from build123d import *

# Parameters (mm, degrees)
SKETCH_3_R          = 3
EXTRUDE_3_DEPTH     = 3
CUT_EXTRUDE_1_DEPTH = 232.050692133


with BuildPart() as part:
    # 草图3 → 凸台-拉伸3 (new body)
    with BuildSketch(Plane(origin=(0, 0, 0), x_dir=(1, 0, 0), z_dir=(0, 1, 0))):
        with BuildLine():
            Line((41.250352709, 37.437096955), (2.1711222, 37.437096955))
            ThreePointArc((2.1711222, 37.437096955), (-37.245354745, -4.362745688), (10.764053756, -35.921931278))
            Line((10.764053756, -35.921931278), (102.964763311, -8.293867902))
            ThreePointArc((102.964763311, -8.293867902), (111.422798179, -6.156653751), (120.034918159, -4.764738657))
            Line((120.034918159, -4.764738657), (134.438707225, -3.077546548))
            ThreePointArc((134.438707225, -3.077546548), (143.139368882, -2.441523824), (151.862354927, -2.566233988))
            Line((151.862354927, -2.566233988), (154.274717881, -2.706136256))
            ThreePointArc((154.274717881, -2.706136256), (158.623829365, -3.053695832), (162.953641123, -3.590630188))
            Line((162.953641123, -3.590630188), (169.76623366, -4.586797783))
            ThreePointArc((169.76623366, -4.586797783), (178.335042253, -6.22434395), (186.728522391, -8.602479637))
            Line((186.728522391, -8.602479637), (194.174928436, -11.067895146))
            Line((194.174928436, -11.067895146), (206.234258671, -17.125709257))
            ThreePointArc((206.234258671, -17.125709257), (225.560310545, -11.871725652), (222.437509756, 7.910810586))
            Line((222.437509756, 7.910810586), (215.500702076, 12.589746446))
            ThreePointArc((215.500702076, 12.589746446), (200.255076036, 21.040534955), (183.773601289, 26.715561818))
            Line((183.773601289, 26.715561818), (174.440874355, 29.042471985))
            ThreePointArc((174.440874355, 29.042471985), (165.892131299, 30.781733417), (157.22433217, 31.769304384))
            Line((157.22433217, 31.769304384), (111.006826453, 35.001147214))
            ThreePointArc((111.006826453, 35.001147214), (76.149849411, 36.827923974), (41.250352709, 37.437096955))
        make_face()
        with Locations(Location((212.967480872, -3.721839712, 0), (0, 0, 270))):
            Circle(SKETCH_3_R, mode=Mode.SUBTRACT)
    extrude(amount=EXTRUDE_3_DEPTH)

    # 草图4 → 切除-拉伸1 (cut, through all)
    with BuildSketch(Plane(origin=(0, 3, 0), x_dir=(1, 0, 0), z_dir=(0, 1, 0))):
        with BuildLine():
            ThreePointArc((136.159607467, 33.242293427), (180.670295505, 25.248626767), (222.437509756, 7.910810586))
            Line((222.437509756, 7.910810586), (215.500702076, 12.589746446))
            ThreePointArc((215.500702076, 12.589746446), (200.255076036, 21.040534955), (183.773601289, 26.715561818))
            Line((183.773601289, 26.715561818), (174.440874355, 29.042471985))
            ThreePointArc((174.440874355, 29.042471985), (165.892131299, 30.781733417), (157.22433217, 31.769304384))
            Line((157.22433217, 31.769304384), (136.159607467, 33.242293427))
        make_face()
    extrude(amount=-CUT_EXTRUDE_1_DEPTH, mode=Mode.SUBTRACT)


solid = part.part
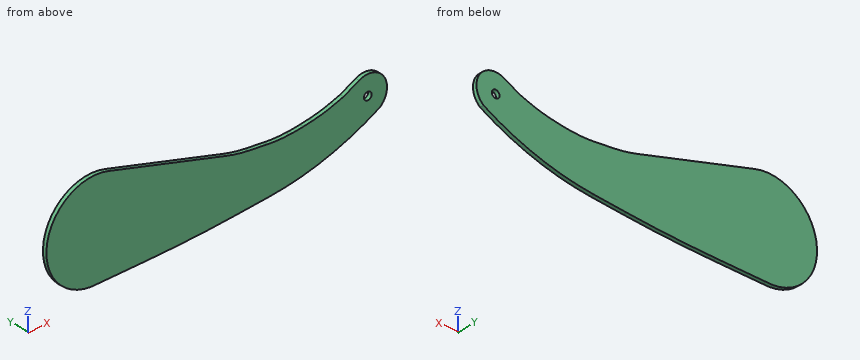
Verification items for the finished model (mm, model axes). Round coordinates to 2 decimals unless told otherwise and drop trailing zeros. Loops run counter-clockwise (first coordinate to the right, second up) from the corner with the lowest first, then second, coordinate; pieces in that order, holes last. Notation, with made-up numbers: (62, 82) - (72, 82) arc R16 ccw to (72, 95) - close; hole circle Ø6 at (10.25, -4). An arc over 180 degrees is marked (long way). Use a Markdown table: item, result. Add a question column.
1. Section check A-A, the plane y = 0.8. Record the boundary of the cut face in (x, z).
2. Section check C-C, the plane z = 26. Record the boundary of the cut face in (x, y), plus the area to 3 significant figures.
3. Thickness scan on probe 1 along Z at (x, y) = (126, 2.6); probe 2 along X at (y, z) = (2.75, -10.5); probe 3 along Z at (x, y) = (2, 0.35). Record the ranges inside material, lowest first. Write a range as [from, to].
4. Section check B-B, the plane x = 57.5. Record the boundary of the cut face in (y, z).
5. Gauge pin test, flat ends, axial feed: pin 1 (12 mm diameter, centred on x = 199.5, z = 24, fed in from +Y); pin 2 (1 mm diameter, centred on y = 1.5, z = 12.5, fed in from +X); pin 3 (1 mm diameter, centred on x = 117.5, y = 2, fed in from -Z); pin 4 (1.5 mm diameter, centred on x = -4, y = 0.5, fed in from +Z). Record the tip position at first contact, or that the pin passes through.
Checks:
| question | item | result |
|---|---|---|
| 1 | outline | (2.17, -37.44) - (41.25, -37.44) arc R1000 ccw to (111.01, -35) - (136.16, -33.24) arc R210 ccw to (222.44, -7.91) arc R15 ccw to (206.23, 17.13) - (194.17, 11.07) - (186.73, 8.6) arc R100 cw to (169.77, 4.59) - (162.95, 3.59) arc R100 cw to (154.27, 2.71) - (151.86, 2.57) arc R100 cw to (134.44, 3.08) - (120.03, 4.76) arc R100 cw to (102.96, 8.29) - (10.76, 35.92) arc R37.5 ccw (long way) to start; hole circle Ø6 at (212.97, 3.72) |
| 2 | outline | (-27.02, 0) - (43.88, 0) - (43.88, 3) - (-27.02, 3) - close |
| 2 | area | 213 mm^2 |
| 3 | probe 1 | z = [-33.95, 4.07] |
| 3 | probe 2 | x = [-36, 217.56] |
| 3 | probe 3 | z = [-37.45, 37.45] |
| 4 | outline | (0, -37.31) - (3, -37.31) - (3, 21.92) - (0, 21.92) - close |
| 5 | pin 1 | passes through |
| 5 | pin 2 | stops at x = 225.48 |
| 5 | pin 3 | stops at z = -34.58 |
| 5 | pin 4 | stops at z = 37.36 |
